from build123d import *

# Parameters (mm, degrees)
SKETCH1_W           = 80
SKETCH1_H           = 280
BOSS_EXTRUDE1_DEPTH = 10
SKETCH6_R           = 5
CUT_EXTRUDE3_DEPTH  = 10


with BuildPart() as part:
    # Sketch1 → Boss-Extrude1 (new body)
    with BuildSketch(Plane.XY):
        Polygon((-90, -160), (-70, -160), (-70, -240), (90, -240), (90, 240), (-90, 240), align=None)
        Rectangle(SKETCH1_W, SKETCH1_H, mode=Mode.SUBTRACT)
    extrude(amount=BOSS_EXTRUDE1_DEPTH)

    # Sketch6 → Cut-Extrude3 (cut)
    with BuildSketch(Plane.XY.offset(10)):
        with Locations((-50, -220)):
            Circle(SKETCH6_R)
        with Locations((-30, -200)):
            Circle(SKETCH6_R)
        with Locations(Location((70, -220, 0), (0, 0, 180))):
            Circle(SKETCH6_R)
        with Locations(Location((50, -200, 0), (0, 0, 180))):
            Circle(SKETCH6_R)
        with Locations((-80, 230)):
            Circle(SKETCH6_R)
        with Locations((80, 230)):
            Circle(SKETCH6_R)
        with Locations((-80, -80)):
            Circle(SKETCH6_R)
        with Locations((-65, -140)):
            Circle(SKETCH6_R)
    extrude(amount=-CUT_EXTRUDE3_DEPTH, mode=Mode.SUBTRACT)


solid = part.part
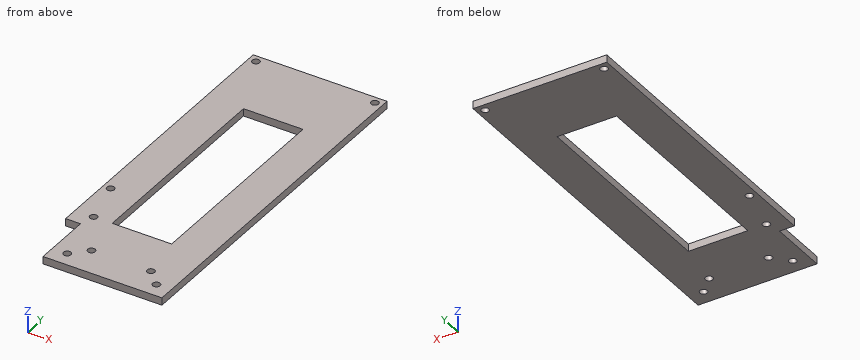
Part model, mm, in its own coordinate system. Give positions to 0.01 mm unless a question says otherwise; leave off trailing zeros. Loops run counter-clockwise (first coordinate to the right, second up) from the corner with the lowest first, then second, coordinate; pieces in that order, holes last. Notation, with made-up numbers: M -38,21 L 13,21 A19 cw 13,31 Z; hole C 5,28.5 d10. An arc over 180 degrees is marked long. Put each result on its own line as item: value. Start each with the question number.
1) Saw through at D-D (z = 1.75). State how many separate pieces and enclosed holes the cut face has, then the cut area to 3 significant figures.
2) Flat gauge pins, fed straight in: pin 1 (3 mm diameter, centred on y = -194.5, z = 6.5, fed in from -X); pin 2 (5 mm diameter, centred on x = -83, z = 5.5, fed in from -Y). Where does each tip first touch, or does it go through?
3) Probe probe 1 along Y at (x, z) = (-80, 6.25); probe 2 along X at (y, z) = (131.5, 4.25); probe 3 along Y at (x, z) = (39, 2.25). List the from-to ranges inside material, lowest first.
4) Saw through at C-C (x = 80). List the corners of the cut face in (y, z).
5) Saw through at A-A (x = -30). List the corners of the cut face in (y, z), then the cut area to 3 significant figures.
6) Saw through at B-B (y = -220). List the corners of the cut face in (x, z), then the cut area to 3 significant figures.
Numbers:
1. separate pieces: 1
1. enclosed holes: 9
1. area: 61,800 mm^2
2. pin 1: x = -70
2. pin 2: y = -160
3. probe 1: -160 to -85, -75 to 225, 235 to 240
3. probe 2: -90 to -40, 40 to 90
3. probe 3: -240 to -140, 140 to 240
4. outline: M -240,0 L 225,0 L 225,10 L -240,10 Z; M 235,0 L 240,0 L 240,10 L 235,10 Z
5. outline: M -240,0 L -205,0 L -205,10 L -240,10 Z; M -195,0 L -140,0 L -140,10 L -195,10 Z; M 140,0 L 240,0 L 240,10 L 140,10 Z
5. area: 1,900 mm^2
6. outline: M -70,0 L -55,0 L -55,10 L -70,10 Z; M -45,0 L 65,0 L 65,10 L -45,10 Z; M 75,0 L 90,0 L 90,10 L 75,10 Z
6. area: 1,400 mm^2
